```python
from build123d import *

# Parameters (mm, degrees)
F0_W     = 200
F0_H     = 100
F0_R     = 22.7241513298
F0_R_2   = 21.9586845422
F1_DEPTH = 25
F2_DEPTH = 200
F3_SIZE  = 20
F4_F1_R  = 5
F4_F2_R  = 5
F4_F3_R  = 5
F4_F4_R  = 5
F4_F5_R  = 5
F4_F6_R  = 5
F4_F7_R  = 5


# Not quite as in the source:
# - a feature of the source that left no trace in its solid (it failed there, or was rolled back) is left out


with BuildPart() as f1:
    # F0 (on Front) → F1 (new body)
    with BuildSketch(Plane.XZ):
        with Locations((-13.0278225988, -29.689514604)):
            Rectangle(F0_W, F0_H)
        with Locations((-70.3068226576, -29.689514604)):
            Circle(F0_R, mode=Mode.SUBTRACT)
        with Locations((44.6292310953, -29.689514604)):
            Circle(F0_R_2, mode=Mode.SUBTRACT)
    extrude(amount=F1_DEPTH)

    # F0 (on Front) → F2 (join)
    with BuildSketch(Plane.XZ):
        with Locations((44.6292310953, -29.689514604)):
            Circle(F0_R_2)
        with Locations((-70.3068226576, -29.689514604)):
            Circle(F0_R)
    extrude(amount=F2_DEPTH)

    # F3
    f3_edges = [f1.edges().sort_by_distance(p)[0] for p in [
        (-13.027823, -25, 20.310485),
    ]]
    chamfer(f3_edges, length=F3_SIZE)

    # F4: fillet of radius 5 on 11 edges, made by hand

    # F4_f1
    f4_f1_edges = [f1.edges().sort_by_distance(p)[0] for p in [
        (-13.0278225988, -5, 20.310485396),
    ]]
    fillet(f4_f1_edges, radius=F4_F1_R)

    # F4_f2
    f4_f2_edges = [f1.edges().sort_by_distance(p)[0] for p in [
        (-13.0278225988, -25, 0.310485396),
    ]]
    fillet(f4_f2_edges, radius=F4_F2_R)

    # F4_f3
    f4_f3_edges = [f1.edges().sort_by_distance(p)[0] for p in [
        (-13.0278225988, -25, -79.689514604),
    ]]
    fillet(f4_f3_edges, radius=F4_F3_R)

    # F4_f4
    f4_f4_edges = [f1.edges().sort_by_distance(p)[0] for p in [
        (-93.0309739873, -25, -29.689514604),
    ]]
    fillet(f4_f4_edges, radius=F4_F4_R)

    # F4_f5
    f4_f5_edges = [f1.edges().sort_by_distance(p)[0] for p in [
        (22.6705465531, -25, -29.689514604),
    ]]
    fillet(f4_f5_edges, radius=F4_F5_R)

    # F4_f6
    f4_f6_edges = [f1.edges().sort_by_distance(p)[0] for p in [
        (86.9721774012, -25, -38.2250485099),
    ]]
    fillet(f4_f6_edges, radius=F4_F6_R)

    # F4_f7
    f4_f7_edges = [f1.edges().sort_by_distance(p)[0] for p in [
        (-113.0278225988, -25, -38.2250485099),
    ]]
    fillet(f4_f7_edges, radius=F4_F7_R)


solid = f1.part
```
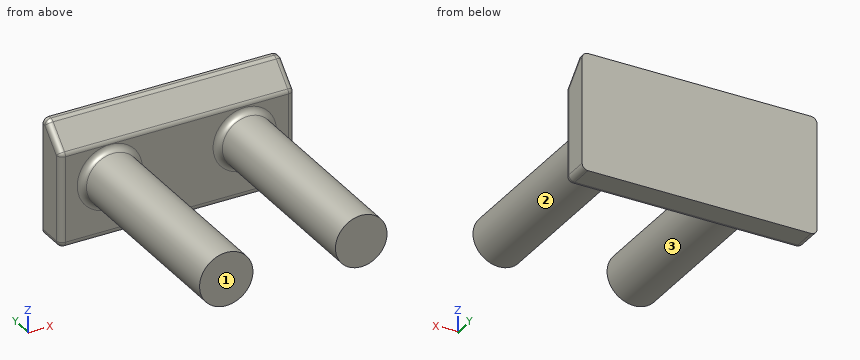
CAD build for the part. Positions are in the model's coordinates, mm. Face numbers are marked on the shaded views. Coordinates: 2 decimals unless noted, no trailing zeros. Order: outer loops, then holes, each group sorted by start corner. A loop starts at its lowest first (then second) coordinate and runs counter-clockwise, first axis right, second up. Notation, with made-up numbers: M 66.5,-5.5 L 88.5,-5.5 A30 cw 88.5,17.5 Z; hole C 7.5,85.25 d8. An arc over 180 degrees is marked long. Write each question's results on one line, items separated by ' | '. Start each with the question number.
Q1. Cut at A-A (x = -27). List the corners of the cut face in (y, z), then the cut area to 3 significant figures.
Q2. Flat gauge pins, fed straight in: P1, Ø2, axis at y = -140.5, z = -38, coming from the +X side; P2, Ø6, axis at x = -25, z = -19, coming from the -Y side; P3, Ø10, axis at y = -70.5, z = -7, coming from the -X side; P4, Ø10, axis at x = -41, y = -77, coming from the -Z side. Where does each tip first touch, or does it go through?
Q3. Cut at B-B (y = -61). List the corners of the cut face in (x, z).
Q4. Drill centre lines: probe 1 along X at (y, z) = (-109, -29); probe 2 along Z at (x, y) = (-70.5, -173.5); probe 3 along Y at (x, z) = (-13, -47.5). Where is each one in solid material? Low to high. Write a range as from..to.
Q5. Pull direction X, two halves, no side cores. Call the marked faces 1, 2 and 3: +X half, -X half, draft (parallel to the pull), parting line (faces both ways), or undercut.
Found:
1) outline: M -25,-74.69 A5 ccw -20,-79.69 L 0,-79.69 L 0,20.31 L -2.93,20.31 A5 ccw -6.46,18.85 L -23.54,1.77 A5 ccw -25,-1.76 Z | area: 2,290 mm²
2) P1: x = 65.34 | P2: y = -25 | P3: x = -84.57 | P4: through
3) outline: C -70.31,-29.69 d45.45; C 44.63,-29.69 d43.92
4) probe 1: -93.02..-47.59, 22.68..66.58 | probe 2: -52.41..-6.97 | probe 3: -25..0
5) face 1: draft | face 2: undercut | face 3: undercut
